from build123d import *

# Parameters (mm, degrees)
SKETCH_4_R      = 32
SKETCH_4_R_2    = 27.5
EXTRUDE_1_DEPTH = 45
CHAMFER_1_SIZE  = 3.2875


with BuildPart() as part:
    # Эскиз1 → Повернуть1 (revolve)
    with BuildSketch(Plane.XY):
        Polygon((-125, 27.5), (-80, 27.5), (0, 17.5), (0, 12.5), (-77.272727273, 12.5), (-125, 25), align=None)
    revolve(axis=Axis((0, 0, 0), (-1, 0, 0)))

    # Эскиз4 → Бобышка-Вытянуть1 (add)
    with BuildSketch(Plane.ZY.offset(125)):
        Circle(SKETCH_4_R)
        Circle(SKETCH_4_R_2, mode=Mode.SUBTRACT)
    extrude(amount=-EXTRUDE_1_DEPTH)

    # Фаска1
    chamfer_1_edges = [part.edges().sort_by_distance(p)[0] for p in [
        (-125, 0, -32),
    ]]
    chamfer(chamfer_1_edges, length=CHAMFER_1_SIZE)


solid = part.part
Geometry: final body of the model. Coordinates: model frame, mm. A direction names the side the tool comes from. Coordinates: 2 decimals unless noted, no trailing zeros. Write each loop counter-clockwise with the first axis right and the second up, starting at its lowest first coordinate (ties: lowest second). Pieces come first, ordered by that corner, then holes. Notation, with made-up numbers: (-36, 40.5) - (8, 40.5) arc R22 cw to (8, 62.5) - close; hole circle Ø1 at (56, -29.5). An arc over 180 degrees is marked (long way). Return JSON: item names as keys, results as strings.
Item 1: Reachability of faces 1 (the face through (-125, 24, -9)), 2 (the face through (-80, 24, 14)) from +Z, -Z, +X, -X, +Y, -Y: full face, straight path, thin tool, end or side. Return the list, or none.
Completed:
{"face 1": "+Z, -Z, -X, +Y, -Y", "face 2": "+X"}
Item 2: Section query C-C (x = -101.5). Output: boundary loops of the cut face in (y, z), and give its area (3 significant figures).
Completed:
{"outline": "circle Ø64 at (0, 0); hole circle Ø37.69 at (0, 0)", "area": "2,100 mm2"}
Item 3: Section query D-D (x = -88). Output: boundary loops of the cut face in (y, z), and give its area (3 significant figures).
Completed:
{"outline": "circle Ø64 at (0, 0); hole circle Ø30.62 at (0, 0)", "area": "2,480 mm2"}
Item 4: Line query: L1, parallel to Z at x = -49.5, y = 0; L2, parallel to Y at x = -70.5, z = 1; L3, parallel to Y at x = -15, z = 0 (3 decimals). Output: solid intervals per line, ascending.
Completed:
{"L1": "z = -23.69 to -12.5, 12.5 to 23.69", "L2": "y = -26.29 to -12.46, 12.46 to 26.29", "L3": "y = -19.375 to -12.5, 12.5 to 19.375"}
Item 5: Pull-direction query (Z, two-part tool) for faces 3 (the face through (0, 11, 8)), 4 (the face through (-39.177, 11.923, -3.755)), 5 (the face through (-101.15, -31.24, -6.94)); classes: +Z half, -Z half, draft (parallel to the pull), parting line (faces both ways), or undercut.
Completed:
{"face 3": "draft", "face 4": "undercut", "face 5": "parting line"}
Item 6: Pin query (flat end, axial travel): pin 1 Ø1.5 at (x, y) = (-74.5, 23) entering from -Z; pin 2 Ø2 at (y, z) = (23, -21) entering from -X; pin 3 Ø10 at (x, y) = (-30, -15) entering from -Z. Return the tip coordinate at first contact, or that it passes through.
Completed:
{"pin 1": "stops at z = -14.97", "pin 2": "stops at x = -123.57", "pin 3": "stops at z = -18.84"}
Item 7: Section query A-A (y = 0). Output: boundary loops of the cut face in (x, z), and give its area (3 significant figures).
Completed:
{"outline": "(-125, -28.71) - (-121.71, -32) - (-80, -32) - (-80, -27.5) - (0, -17.5) - (0, -12.5) - (-77.27, -12.5) - (-125, -25) - close; (-125, 25) - (-77.27, 12.5) - (0, 12.5) - (0, 17.5) - (-80, 27.5) - (-80, 32) - (-121.71, 32) - (-125, 28.71) - close", "area": "2,750 mm2"}
